Here's how the part is built. I have some questions about the finished solid (model axes, mm). A direction names the side the tool comes from. Coordinates: 2 decimals unless noted, no trailing zeros. Write each loop counter-clockwise with the first axis right and the second up, starting at its lowest first coordinate (ties: lowest second). Pieces come first, ordered by that corner, then holes.
(1) For pin 1 Ø1 at (x, y) = (-3.5, 0) entering from +Z, with a flat end and sliding along its axis, tell me the tip position at first contact or that it passes through.
(2) Which directions (+Z, -Z, +X, -X, +Y, -Y) give clear straight access to the entire face, cutting with the end or side of a thin tool? Please do faces 1 (the flat face through (3, 0, -9.9)), 2 (the flat face through (4, 0, 0.1)), 3 (the flat face through (-28, 0, -5)).
(3) Imagine slicing it at A-A, the plane y = 0.75. List the corners of the cut face in (x, z) for me.
(4) Imagine slicing it at B-B, the plane x = 28. List the corners of the cut face in (y, z) for me, plus the area to 3 significant figures.
(5) Please list where these lines run through material, in increasing order: probe 1 along X at (y, z) = (-0.4, -11.5); probe 2 along Z at (x, y) = (8.5, 0.5); probe 3 along Z at (x, y) = (40, -0.2).
(6) Thinking about a two-plate mould opening in Z: for faces 4 (the flat face through (49.565, -0.021, -2.435)), 5 (the cylindrical face through (-31.075, -0.021, 4.885)), 6 (the flat face through (6, -1.5, -5)), which applies, released by +Z, released by -Z, zero draft, split by the parting line, or undercut?
(7) Imagine slicing it at C-C, the plane z = -14.5. List the corners of the cut face in (x, y) for me.
```python
from build123d import *

# Parameters (mm, degrees)
F1_DEPTH = 1.5


with BuildPart() as f1:
    # F0 (on Front) → F1 (new body, symmetric)
    with BuildSketch(Plane.XZ):
        with BuildLine():
            ThreePointArc((-23.4997773468, 1.5999988765), (-31.1817578622, 4.7819793918), (-27.9997773468, -2.9000011235))
            ThreePointArc((-27.9997773468, -2.9000011235), (-24.8177968315, -1.5819816389), (-23.4997773468, 1.5999988765))
        make_face()
        with BuildLine():
            ThreePointArc((-27.9997773468, 0.0999988765), (-29.0604375186, 2.6606590482), (-26.4997773468, 1.5999988765))
            ThreePointArc((-26.4997773468, 1.5999988765), (-26.9391171751, 0.5393387047), (-27.9997773468, 0.0999988765))
        make_face(mode=Mode.SUBTRACT)
        with BuildLine():
            ThreePointArc((-23.4997773468, 1.5999988765), (-24.8177968315, -1.5819816389), (-27.9997773468, -2.9000011235))
            Line((-27.9997773468, -2.9000011235), (-27.9997773468, -4.9000011235))
            Line((-27.9997773468, -4.9000011235), (-27.9997773468, -6.9000011235))
            ThreePointArc((-27.9997773468, -6.9000011235), (-24.8177968315, -8.2180206082), (-23.4997773468, -11.4000011235))
            Line((-23.4997773468, -11.4000011235), (-23.4997773468, -9.9000011235))
            Line((-23.4997773468, -9.9000011235), (-23.4997773468, -4.9000011235))
            Line((-23.4997773468, -4.9000011235), (-23.4997773468, 0.0999988765))
            Line((-23.4997773468, 0.0999988765), (-23.4997773468, 1.5999988765))
        make_face()
        Polygon((30.4666368291, 0.0999988765), (-23.4997773468, 0.0999988765), (-23.4997773468, -4.9000011235), (-23.4997773468, -9.9000011235), (30.4666368291, -9.9000011235), (68.1362532328, -4.9000011235), align=None)
        with BuildLine():
            ThreePointArc((-23.4997773468, -11.4000011235), (-24.8177968315, -8.2180206082), (-27.9997773468, -6.9000011235))
            ThreePointArc((-27.9997773468, -6.9000011235), (-31.1817578622, -14.5819816389), (-23.4997773468, -11.4000011235))
        make_face()
        with BuildLine():
            ThreePointArc((-26.4997773468, -11.4000011235), (-29.0604375186, -12.4606612953), (-27.9997773468, -9.9000011235))
            ThreePointArc((-27.9997773468, -9.9000011235), (-26.9391171751, -10.3393409518), (-26.4997773468, -11.4000011235))
        make_face(mode=Mode.SUBTRACT)
    extrude(amount=F1_DEPTH, both=True)


solid = f1.part
```
Recorded:
1. pin 1: stops at z = 0.1
2. face 1: -Z, +X, +Y, -Y
2. face 2: +Z, +X, +Y, -Y
2. face 3: -X, +Y, -Y
3. outline: (-28, -6.9) arc R4.5 ccw (long way) to (-23.5, -11.4) - (-23.5, -9.9) - (30.47, -9.9) - (68.14, -4.9) - (30.47, 0.1) - (-23.5, 0.1) - (-23.5, 1.6) arc R4.5 ccw (long way) to (-28, -2.9) - close; hole circle Ø3 at (-28, -11.4); hole circle Ø3 at (-28, 1.6)
4. outline: (-1.5, -9.9) - (1.5, -9.9) - (1.5, 0.1) - (-1.5, 0.1) - close
4. area: 30.0 mm2
5. probe 1: x = -32.5 to -29.5, -26.5 to -23.5
5. probe 2: z = -9.9 to 0.1
5. probe 3: z = -8.63 to -1.17
6. face 4: released by +Z
6. face 5: undercut
6. face 6: zero draft
7. outline: (-31.26, -1.5) - (-24.74, -1.5) - (-24.74, 1.5) - (-31.26, 1.5) - close
